Check sheet for the modelled part. Datum: model origin and axes. Units: mm. Face numbers are marked on the shaded views. A direction names the side the tool comes from. Coordinates: 2 decimals unless noted, no trailing zeros. Loops run counter-clockwise (first coordinate to the right, second up) from the corner with the lowest first, then second, coordinate; pieces in that order, holes last. Notation, with made-up numbers: M -12,21 L 5,21 A20 ccw 5,55 Z; hole C 22.5,-38.75 d5. An arc over 180 degrees is marked long. Return JSON: item names as keys, results as strings.
from build123d import *

# Parameters (mm, degrees)
SKETCH1_W           = 93.98
SKETCH1_H           = 19.05
BOSS_EXTRUDE1_DEPTH = 2.6289
SKETCH2_W           = 93.98
SKETCH2_H           = 25.4
BOSS_EXTRUDE2_DEPTH = 5.2578
FILLET6_R           = 4.572
FILLET7_R           = 4.572
FILLET8_R           = 1.524
FILLET9_R           = 2.54
FILLET10_R          = 2.54


with BuildPart() as part:
    # Sketch1 → Boss-Extrude1 (new body, symmetric)
    with BuildSketch(Plane.XY):
        Rectangle(SKETCH1_W, SKETCH1_H)
    extrude(amount=BOSS_EXTRUDE1_DEPTH, both=True)

    # Sketch2 → Boss-Extrude2 (add)
    with BuildSketch(Plane(origin=(0, 9.525, 0), x_dir=(1, 0, 0), z_dir=(0, 1, 0))):
        with Locations((0, 10.0711)):
            Rectangle(SKETCH2_W, SKETCH2_H)
    extrude(amount=BOSS_EXTRUDE2_DEPTH)

    # Fillet6
    fillet6_edges = [part.edges().sort_by_distance(p)[0] for p in [
        (-46.99, -9.525, 0),
    ]]
    fillet(fillet6_edges, radius=FILLET6_R)

    # Fillet7
    fillet7_edges = [part.edges().sort_by_distance(p)[0] for p in [
        (46.99, -9.525, 0),
    ]]
    fillet(fillet7_edges, radius=FILLET7_R)

    # Fillet8
    fillet8_edges = [part.edges().sort_by_distance(p)[0] for p in [
        (0, 14.7828, 2.6289),
    ]]
    fillet(fillet8_edges, radius=FILLET8_R)

    # Fillet9
    fillet9_edges = [part.edges().sort_by_distance(p)[0] for p in [
        (-46.99, 12.1539, -22.7711),
    ]]
    fillet(fillet9_edges, radius=FILLET9_R)

    # Fillet10
    fillet10_edges = [part.edges().sort_by_distance(p)[0] for p in [
        (46.99, 12.1539, -22.7711),
    ]]
    fillet(fillet10_edges, radius=FILLET10_R)


solid = part.part
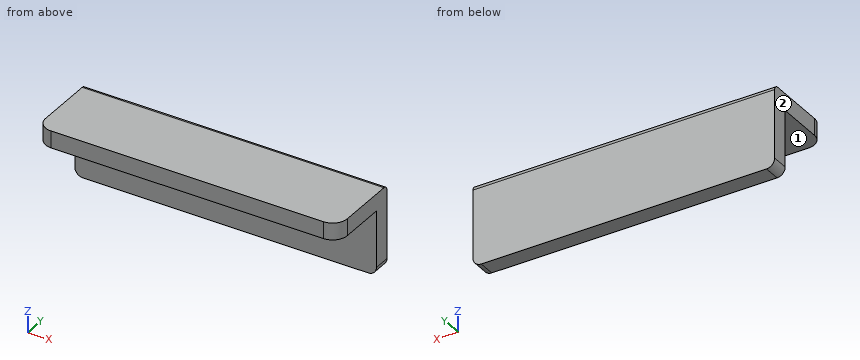
1) Go/stop test with a flat-tipped pin: pin 1 Ø5 at (x, z) = (-3, -19.5) entering from -Y (3 decimals). Record where the tip stops, or that it passes through.
Answers:
{"pin 1": "y = 9.525"}
2) Section check C-C on z = -11. Record the cut outline in (x, y) (3 decimals).
Answers:
{"outline": "M -46.99,9.525 L 46.99,9.525 L 46.99,14.783 L -46.99,14.783 Z"}
3) Scan lines: line 1 along Z through (x, y) = (37.5, 9); line 2 along Y through (x, z) = (-4.5, -17.5) (3 decimals). Record each from-to range of solid material in increasing order. Write a range as [from, to].
Answers:
{"line 1": "[-2.63, 2.63]", "line 2": "[9.525, 14.783]"}
4) Set-up check for the marked faces 1 and 2: record each of +Z, -Z, +X, -X, +Y, -Y from which the full face is reachable in a straight line by a thin tool's end or side.
Answers:
{"face 1": "-Z, +X, -X, -Y", "face 2": "+Z, -Z, -X, +Y, -Y"}
5) Section check B-B on y = 0.5. Record the cut outline in (x, z), then the cut area to 3 significant figures.
Answers:
{"outline": "M -46.99,-2.63 L 46.99,-2.63 L 46.99,2.63 L -46.99,2.63 Z", "area": "494 mm²"}
6) Section check A-A on x = -15.5. Record the cut outline in (y, z) (3 decimals).
Answers:
{"outline": "M -9.525,-2.629 L 9.525,-2.629 L 9.525,-22.771 L 14.783,-22.771 L 14.783,1.105 A1.524 ccw 13.259,2.629 L -9.525,2.629 Z"}
